Model file for the job. Use its own axes, mm. A direction names the side the tool comes from. Coordinates: 2 decimals unless noted, no trailing zeros. Loops run counter-clockwise (first coordinate to the right, second up) from the corner with the lowest first, then second, coordinate; pieces in that order, holes last.
from build123d import *

# Parameters (mm, degrees)
F0_W     = 107.95
F0_H     = 19.05
F1_DEPTH = 3.175
F2_W     = 3.175
F2_H     = 19.05
F3_DEPTH = 81.28
F4_SIZE  = 5.08
F5_R     = 7.62
F6_DEPTH = 107.95
F7_R     = 5.906651
F7_R_2   = 6.296928
F8_DEPTH = 3.175


with BuildPart() as f1:
    # F0 (on Top) → F1 (new body)
    with BuildSketch(Plane.XY):
        Rectangle(F0_W, F0_H)
    extrude(amount=-F1_DEPTH)

    # F2 (on Top) → F3 (join)
    with BuildSketch(Plane.XY):
        with Locations((-52.3875, 0)):
            Rectangle(F2_W, F2_H)
        with Locations((52.3875, 0)):
            Rectangle(F2_W, F2_H)
    extrude(amount=F3_DEPTH)

    # F4
    f4_edges = [f1.edges().sort_by_distance(p)[0] for p in [
        (52.3875, -9.525, 81.28),
        (52.3875, 9.525, 81.28),
        (-52.3875, -9.525, 81.28),
        (-52.3875, 9.525, 81.28),
    ]]
    chamfer(f4_edges, length=F4_SIZE)

    # F5 (on face) → F6 (cut, through all)
    with BuildSketch(Plane(origin=(-53.975, 0, 0), x_dir=(0, -1, 0), z_dir=(-1, 0, 0))):
        with Locations((0, 52.705)):
            Circle(F5_R)
    extrude(amount=-F6_DEPTH, mode=Mode.SUBTRACT)

    # F7 (on face) → F8 (cut, through all)
    with BuildSketch(Plane.XY):
        with Locations((-30.449122, 0)):
            Circle(F7_R)
        with Locations((30.510878, 0)):
            Circle(F7_R_2)
    extrude(amount=-F8_DEPTH, mode=Mode.SUBTRACT)


solid = f1.part
Q1. Flat gauge pin, fed straight in: P1, Ø4, axis at x = 37.5, y = 0, coming from the +Z side. Where does the tip first touch, or does it go through?
Answers:
P1: stops at z = 0
Q2. Mould opens along X. For faces 3 (the flat face through (-1, 0, 0)), 4 (the flat face through (52.365, 7.021, 78.704)), 5 (the flat face through (53.975, 0, 40)) say: +X half, -X half, draft (parallel to the pull), parting line (faces both ways), or undercut.
Answers:
face 3: undercut
face 4: draft
face 5: +X half
Q3. Slice it at B-B (z = 16). List the corners of the cut face in (x, y) (3 decimals).
Answers:
outline: (-53.975, -9.525) - (-50.8, -9.525) - (-50.8, 9.525) - (-53.975, 9.525) - close; (50.8, -9.525) - (53.975, -9.525) - (53.975, 9.525) - (50.8, 9.525) - close
Q4. Which spindle directions (+Z, -Z, +X, -X, +Y, -Y) get a long thin tool onto all of the face, cutting with end or side? Do faces 1 (the flat face through (-50.8, 0, 40)), 2 (the flat face through (-52.41, -6.949, 78.776)). Say none if no direction does.
Answers:
face 1: +Z, +Y, -Y
face 2: +Z, +X, -X, -Y
Q5. Slice it at A-A (y = -1.5). List the corners of the cut face in (x, z) (3 decimals).
Answers:
outline: (-53.975, -3.175) - (-36.162, -3.175) - (-36.162, 0) - (-50.8, 0) - (-50.8, 45.234) - (-53.975, 45.234) - close; (-53.975, 60.176) - (-50.8, 60.176) - (-50.8, 81.28) - (-53.975, 81.28) - close; (-24.736, -3.175) - (24.395, -3.175) - (24.395, 0) - (-24.736, 0) - close; (36.627, -3.175) - (53.975, -3.175) - (53.975, 45.234) - (50.8, 45.234) - (50.8, 0) - (36.627, 0) - close; (50.8, 60.176) - (53.975, 60.176) - (53.975, 81.28) - (50.8, 81.28) - close
Q6. Slice it at D-D (x = 11.5). List the corners of the cut face in (y, z) (3 decimals), and give its area (3 significant figures).
Answers:
outline: (-9.525, -3.175) - (9.525, -3.175) - (9.525, 0) - (-9.525, 0) - close
area: 60.5 mm2
Q7. Drill centre lines: line 1 (X direction, y = 0.75, z = 77.5) (3 decimals); line 2 (Z direction, x = 19.5, y = -7) (3 decimals). Where is each one in solid material? Low to high.
Answers:
line 1: x = -53.975 to -50.8, 50.8 to 53.975
line 2: z = -3.175 to 0
Q8. Slice it at C-C (z = 56). List the corners of the cut face in (x, y) (3 decimals), and give its area (3 significant figures).
Answers:
outline: (-53.975, -9.525) - (-50.8, -9.525) - (-50.8, -6.871) - (-53.975, -6.871) - close; (-53.975, 6.871) - (-50.8, 6.871) - (-50.8, 9.525) - (-53.975, 9.525) - close; (50.8, -9.525) - (53.975, -9.525) - (53.975, -6.871) - (50.8, -6.871) - close; (50.8, 6.871) - (53.975, 6.871) - (53.975, 9.525) - (50.8, 9.525) - close
area: 33.7 mm2
